Geometry check sheet. Reference: the model listing, model coordinates, mm. Coordinates: 2 decimals unless noted, no trailing zeros. Write each loop counter-clockwise with the first axis right and the second up, starting at its lowest first coordinate (ties: lowest second). Pieces come first, ordered by that corner, then holes. Notation, with made-up numbers: (74, 30.25) -> (93, 30.25) arc R18 cw to (93, 50.25) -> close; hole circle Ø11 at (47, 65.5). An arc over 180 degrees is marked (long way). Answer as CSV lines item,"result".
Autodesk Inventor part; units mm, degrees
ref_plane "YZ Plane" through (0, 0, 0) normal (1, 0, 0) x (0, 1, 0)
ref_plane "XZ Plane" through (0, 0, 0) normal (0, 1, 0) x (-1, 0, 0)
ref_plane "XY Plane" through (0, 0, 0) normal (0, 0, 1) x (1, 0, 0)
sketch "Sketch1" plane through (0, 0, 0) normal (1, 0, 0) x (0, 1, 0)
  line L0 (-216, 200) -> (216, 200)
  line L1 (216, 200) -> (216, -200)
  line L2 (216, -200) -> (-216, -200)
  line L3 (-216, -200) -> (-216, 200)
  line L4 (-216, 200) -> (216, -200) construction
  line L5 (216, 200) -> (-216, -200) construction
  point P0 (0, 0)
  dimension "d0" = 400
  dimension "d1" = 432
extrude "Extrusion1" add sketch "Sketch1" along normal mid plane 3
sketch "Sketch2" plane through (1.5, 0, 0) normal (1, 0, 0) x (0, 0, -1)
  line L0 (200, 216) -> (-200, 216)
  line L1 (-200, -216) -> (200, -216)
  line L2 (200, -216) -> (200, 216)
  line L3 (200, 166) -> (140, 166)
  line L4 (140, 166) -> (140, 128)
  line L5 (140, 128) -> (-70, 128)
  line L6 (-70, 128) -> (-70, -128)
  line L7 (-70, -128) -> (140, -128)
  line L8 (140, -128) -> (140, -166)
  line L9 (140, -166) -> (200, -166)
  point P0 (0, 0)
  dimension "d6" = 50
  dimension "d7" = 50
  dimension "d8" = 60
  dimension "d9" = 38
  dimension "d10" = 270
extrude "Extrusion2" cut sketch "Sketch2" against normal blind 3
sketch "Sketch3" plane through (-1.5, 0, 0) normal (-1, 0, 0) x (0, 0, 1)
  circle A0 centre (97, -199) radius 3
  circle A1 centre (-3, -199) radius 3
  circle A2 centre (-103, -199) radius 3
  line L0 (-200, -216) -> (200, -216)
  line L1 (200, -216) -> (200, 216)
  point P0 (0, 0)
  dimension "d15" = 6
  dimension "d16" = 6
  dimension "d17" = 6
  dimension "d18" = 17
  dimension "d19" = 103
  dimension "d20" = 100
  dimension "d21" = 100
extrude "Extrusion3" cut sketch "Sketch3" against normal blind 3
mirror "Mirror1" about plane through (0, 0, 0) normal (0, 1, 0) of "Extrusion3"
sketch "Sketch4" plane through (-1.5, 0, 0) normal (-1, 0, 0) x (0, 0, 1)
  circle A0 centre (183, 87) radius 2.5
  circle A1 centre (183, -13) radius 2.5
  circle A2 centre (183, -113) radius 2.5
  point P0 (0, 0)
hole "Hole1" at (-1.5, 87, 183) at (-1.5, -13, 183) at (-1.5, -113, 183) direction (1, 0, 0) diameter 6 depth 14.2 tip angle 118
equation "\"d6\" = d7"
properties part number "HCMUTE-CDT23-KXL_A03" material "PMMA Plastic"
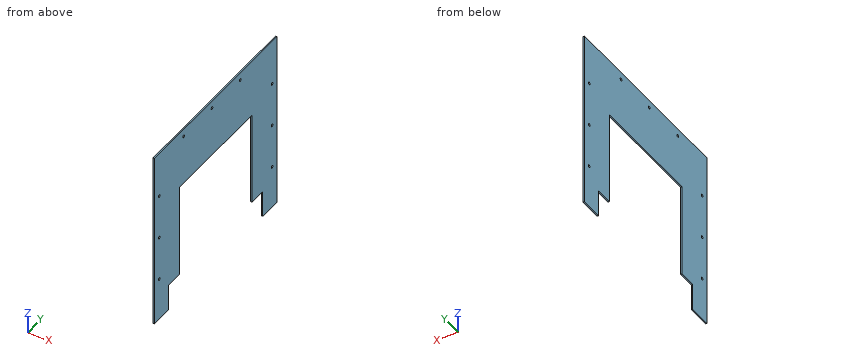
Item 1: Thickness scan on probe 1 along Z at (x, y) = (-0.1, -199); probe 2 along Y at (x, z) = (-1.35, -44); probe 3 along Y at (x, z) = (0.25, 183). Record the ranges inside material, lowest first.
Responses:
probe 1,"z = -200 to -106, -100 to -6, 0 to 94, 100 to 200"
probe 2,"y = -216 to -128, 128 to 216"
probe 3,"y = -216 to -116, -110 to -16, -10 to 84, 90 to 216"
Item 2: Depth check by flat-ended pin: pin 1 Ø5 at (y, z) = (199, -103) entering from -X. Enter the tip coordinate at first touch or a pass-through.
Responses:
pin 1,"passes through"
Item 3: Cross-section at A-A, the plane z = -67. Record the cut outline in (x, y).
Responses:
outline,"(-1.5, -216) -> (1.5, -216) -> (1.5, -128) -> (-1.5, -128) -> close; (-1.5, 128) -> (1.5, 128) -> (1.5, 216) -> (-1.5, 216) -> close"
Item 4: Cross-section at C-C, the plane y = -84. Record the cut outline in (x, z), plus the area to 3 significant figures.
Responses:
outline,"(-1.5, 70) -> (1.5, 70) -> (1.5, 200) -> (-1.5, 200) -> close"
area,"390 mm2"
Item 5: Cross-section at B-B, the plane x = 0.65. Count the separate pieces of the cut face and the enclosed holes in it, plus the area to 3 significant figures.
Responses:
separate pieces,"1"
enclosed holes,"9"
area,"98,900 mm2"
